Geometry check sheet. Reference: drawing and pictorial views, mm from the part's lowest x, y, z. Round coordinates to 2 decimals unless told otherwise and drop trailing zeros. Write each loop counter-clockwise with the first axis right and the second up, starting at its lowest first coordinate (ties: lowest second). Pieces come first, ordered by that corner, then holes. Notation, with made-up numbers: (-10.75, 13) -> (9.25, 13) arc R20 ccw to (9.25, 23) -> close; hole circle Ø2 at (3, 59). An arc over 180 degrees is marked (long way). Write item = value, one per line.
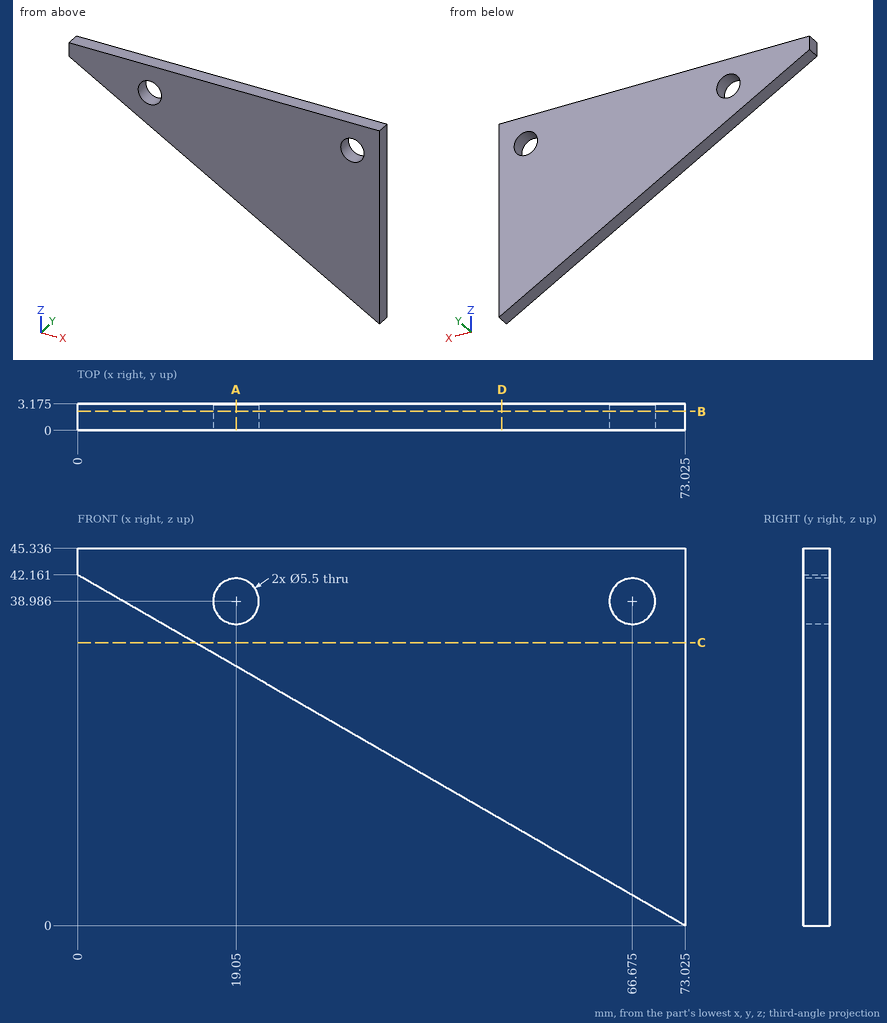
(1) Material ranges on L1, parallel to X at y = 0.85, z = 38.5 (3 decimals); L2, parallel to Z at x = 19.05, y = 2.1; L3, parallel to Z at x = 5.5, y = 0.2, recorded low to high. Write a range as [from, to].
Worked answers:
L1 = [6.341, 16.343], [21.757, 63.968], [69.382, 73.025]
L2 = [31.16, 36.24], [41.74, 45.34]
L3 = [38.99, 45.34]
(2) Sectioned sample at A-A on x = 19.05. Enter the section's corners in (y, z) (3 decimals), then the cut area to 3 significant figures.
Worked answers:
outline = (0, 31.162) -> (3.175, 31.162) -> (3.175, 36.236) -> (0, 36.236) -> close; (0, 41.736) -> (3.175, 41.736) -> (3.175, 45.336) -> (0, 45.336) -> close
area = 27.5 mm²
(3) Sectioned sample at B-B on y = 2.3. Enter the section's corners in (x, z) (3 decimals).
Worked answers:
outline = (0, 42.161) -> (73.025, 0) -> (73.025, 45.336) -> (0, 45.336) -> close; hole circle Ø5.5 at (19.05, 38.986); hole circle Ø5.5 at (66.675, 38.986)
(4) Sectioned sample at D-D on x = 51. Enter the section's corners in (y, z) (3 decimals), then the cut area to 3 significant figures.
Worked answers:
outline = (0, 12.716) -> (3.175, 12.716) -> (3.175, 45.336) -> (0, 45.336) -> close
area = 104 mm²
(5) Sectioned sample at C-C on z = 34. Enter the section's corners in (x, y) (3 decimals), then the cut area to 3 significant figures.
Worked answers:
outline = (14.135, 0) -> (73.025, 0) -> (73.025, 3.175) -> (14.135, 3.175) -> close
area = 187 mm²
